Design review of the part built by this model. Coordinates are the model's own, in mm. A direction names the side the tool comes from. Round coordinates to 2 decimals unless told otherwise and drop trailing zeros. Loops run counter-clockwise (first coordinate to the right, second up) from the corner with the lowest first, then second, coordinate; pieces in that order, holes last. Notation, with made-up numbers: (69, 51.5) - (121, 51.5) arc R24 ccw to (121, 75.5) - close; hole circle Ø8 at (45.25, 11). An arc over 180 degrees is marked (long way). Return JSON: item names as keys, results as strings. Group by question number.
(1) The part is to be moulded in two halves that separate along Y. For faces 1 (the cylindrical face through (400.073, 282.523, 6.036)), 2 (the flat face through (466, 440, 11.906)), say which applies: pulls with the +Y half, pulls with the -Y half, needs draft (parallel to the pull), parting line crosses it, or undercut.
(2) Wall thickness on L1, parallel to X at y = 544, z = 4.5; L2, parallel to X at y = 342.9, z = 6; L3, parallel to Y at x = 745, z = 1: over which ranges is each line inside the solid? List them lowest first. Write a range as [from, to].
(3) We need section A-A, the plane y = 550.5. Write out the cut boundary in (x, z), and give its area (3 significant figures).
(4) We need section B-B, the plane z = 8.5. Write out the cut boundary in (x, y) (3 decimals).
(5) For faces 3 (the cylindrical face through (819.127, 276.277, 6.036)), 4 (the flat face through (466, 440, 0)), list the 3-axis set-ups (+Z, -Z, +X, -X, +Y, -Y) from which the entire face can be reached by the end or side of a thin tool; tool diameter is ignored.
(6) We need section D-D, the plane y = 139. Write out the cut boundary in (x, z), and give its area (3 significant figures).
(7) We need section C-C, the plane x = 629.5. Write out the cut boundary in (y, z).
(8) Clearance check with a flat-ended pin moving along its axis: pin 1 (2 mm diameter, centred on x = 672, z = 6, fed in from -Y). State where the tip first meets the part, or that it passes through.
from build123d import *

# Parameters (mm, degrees)
SKETCH1_W           = 1219.2
SKETCH1_H           = 1778
SKETCH1_R           = 254
SKETCH1_W_2         = 361.95
SKETCH1_H_2         = 361.95
BOSS_EXTRUDE1_DEPTH = 11.90625
SKETCH3_R           = 209.55
CUT_EXTRUDE2_DEPTH  = 12.90625
SKETCH2_W           = 203.2
SKETCH2_H           = 165.1
CUT_EXTRUDE1_DEPTH  = 12.90625
SKETCH5_R           = 3.429
CUT_EXTRUDE4_DEPTH  = 12.90625
LPATTERN2_COUNT     = 3
LPATTERN2_PITCH     = 301.625
SKETCH7_R           = 3.3782
CUT_EXTRUDE6_DEPTH  = 12.90625
SKETCH12_R          = 4.7625
CUT_EXTRUDE7_DEPTH  = 12.90625
SKETCH16_R          = 4.7625
CUT_EXTRUDE10_DEPTH = 12.90625
FILLET2_R           = 6.35
SKETCH19_W          = 1219.2
SKETCH19_H          = 1066.8
CUT_EXTRUDE13_DEPTH = 12.7


with BuildPart() as part:
    # Sketch1 → Boss-Extrude1 (new body)
    with BuildSketch(Plane.XY):
        with Locations((609.6, 889)):
            Rectangle(SKETCH1_W, SKETCH1_H)
        with Locations((330.2, 1473.2)):
            Circle(SKETCH1_R, mode=Mode.SUBTRACT)
        with Locations((609.6, 917.575)):
            Rectangle(SKETCH1_W_2, SKETCH1_H_2, mode=Mode.SUBTRACT)
    extrude(amount=BOSS_EXTRUDE1_DEPTH)

    # Sketch3 → Cut-Extrude2 (cut, through all)
    with BuildSketch(Plane.XY.offset(11.90625)):
        with Locations((609.6, 279.4)):
            Circle(SKETCH3_R)
    extrude(amount=-CUT_EXTRUDE2_DEPTH, mode=Mode.SUBTRACT)

    # Sketch2 → Cut-Extrude1 (cut, through all)
    with BuildSketch(Plane.XY.offset(11.90625)):
        with Locations((609.6, 44.45)):
            Rectangle(SKETCH2_W, SKETCH2_H)
        with Locations((609.6, 514.35)):
            Rectangle(SKETCH2_W, SKETCH2_H)
    extrude(amount=-CUT_EXTRUDE1_DEPTH, mode=Mode.SUBTRACT)

    # Sketch5 → Cut-Extrude4 (cut, through all)
    with BuildSketch(Plane.XY.offset(11.90625)):
        with Locations((609.6, 1714.5)):
            Circle(SKETCH5_R)
    cut_extrude4 = extrude(amount=-CUT_EXTRUDE4_DEPTH, mode=Mode.SUBTRACT)

    # LPattern2: Cut-Extrude4 ×3
    with Locations(*[(0, -i * LPATTERN2_PITCH, 0) for i in range(1, LPATTERN2_COUNT)]):
        add(cut_extrude4, mode=Mode.SUBTRACT)

    # Sketch7 → Cut-Extrude6 (cut, through all)
    with BuildSketch(Plane.XY.offset(11.90625)):
        with Locations((777.605208253, 88.9)):
            Circle(SKETCH7_R)
        with Locations((898.525, 342.9)):
            Circle(SKETCH7_R)
        with Locations((898.525, 215.9)):
            Circle(SKETCH7_R)
    extrude(amount=-CUT_EXTRUDE6_DEPTH, mode=Mode.SUBTRACT)

    # Sketch12 → Cut-Extrude7 (cut, through all)
    with BuildSketch(Plane.XY.offset(11.90625)):
        with Locations((203.2, 1727.2)):
            Circle(SKETCH12_R)
        with Locations((1016, 1727.2)):
            Circle(SKETCH12_R)
    extrude(amount=-CUT_EXTRUDE7_DEPTH, mode=Mode.SUBTRACT)

    # Sketch16 → Cut-Extrude10 (cut, through all)
    with BuildSketch(Plane.XY.offset(11.90625)):
        with Locations((419.1, 1054.1)):
            Circle(SKETCH16_R)
        with Locations((419.1, 787.4)):
            Circle(SKETCH16_R)
        with Locations((800.1, 1054.1)):
            Circle(SKETCH16_R)
        with Locations((800.1, 787.4)):
            Circle(SKETCH16_R)
    extrude(amount=-CUT_EXTRUDE10_DEPTH, mode=Mode.SUBTRACT)

    # Fillet2
    fillet2_edges = [part.edges().sort_by_distance(p)[0] for p in [
        (428.625, 1098.55, 5.953125),
        (428.625, 736.6, 5.953125),
        (790.575, 736.6, 5.953125),
        (790.575, 1098.55, 5.953125),
        (711.2, 596.9, 5.953125),
        (508, 596.9, 5.953125),
        (0, 0, 5.953125),
        (1219.2, 0, 5.953125),
    ]]
    fillet(fillet2_edges, radius=FILLET2_R)

    # Sketch19 → Cut-Extrude13 (cut)
    with BuildSketch(Plane.XY.offset(11.90625)):
        with Locations((609.6, 1244.6)):
            Rectangle(SKETCH19_W, SKETCH19_H)
    extrude(amount=-CUT_EXTRUDE13_DEPTH, mode=Mode.SUBTRACT)


solid = part.part
Solutions:
{
 "1": {"face 1": "undercut", "face 2": "needs draft"},
 "2": {"L1": "[0, 508], [711.2, 1219.2]", "L2": "[0, 409.9], [809.3, 895.15], [901.9, 1219.2]", "L3": "[0, 119.47], [439.33, 711.2]"},
 "3": {"outline": "(0, 0) - (508, 0) - (508, 11.91) - (0, 11.91) - close; (711.2, 0) - (1219.2, 0) - (1219.2, 11.91) - (711.2, 11.91) - close", "area": "12,100 mm^2"},
 "4": {"outline": "(0, 6.35) arc R6.35 ccw to (6.35, 0) - (508, 0) - (508, 96.128) arc R209.55 cw to (508, 462.672) - (508, 590.55) arc R6.35 cw to (514.35, 596.9) - (704.85, 596.9) arc R6.35 cw to (711.2, 590.55) - (711.2, 462.672) arc R209.55 cw to (711.2, 96.128) - (711.2, 0) - (1212.85, 0) arc R6.35 ccw to (1219.2, 6.35) - (1219.2, 711.2) - (0, 711.2) - close; hole circle Ø6.756 at (777.605, 88.9); hole circle Ø6.756 at (898.525, 215.9); hole circle Ø6.756 at (898.525, 342.9)"},
 "5": {"face 3": "+Z, -Z", "face 4": "-Z, +X, -X, +Y, -Y"},
 "6": {"outline": "(0, 0) - (454.04, 0) - (454.04, 11.91) - (0, 11.91) - close; (765.16, 0) - (1219.2, 0) - (1219.2, 11.91) - (765.16, 11.91) - close", "area": "10,800 mm^2"},
 "7": {"outline": "(596.9, 0) - (711.2, 0) - (711.2, 11.91) - (596.9, 11.91) - close"},
 "8": {"pin 1": "y = 596.9"}
}
